```python
from build123d import *

# Parameters (mm, degrees)
SKETCH1_W           = 72
SKETCH1_H           = 42
BOSS_EXTRUDE1_DEPTH = 5
SKETCH2_R           = 1.75
CUT_EXTRUDE1_DEPTH  = 10
D_GAGEMENT_M51_D    = 5.5
SKETCH6_R           = 12.5
CUT_EXTRUDE2_DEPTH  = 42.976183724


with BuildPart() as part:
    # Sketch1 → Boss-Extrude1 (new body)
    with BuildSketch(Plane.XY):
        Rectangle(SKETCH1_W, SKETCH1_H)
    extrude(amount=BOSS_EXTRUDE1_DEPTH)

    # Sketch2 → Cut-Extrude1 (cut)
    with BuildSketch(Plane.XY.offset(5)):
        with Locations((30.475, 15.5)):
            Circle(SKETCH2_R)
        with Locations((30.475, -15.5)):
            Circle(SKETCH2_R)
        with Locations((-0.525, -15.5)):
            Circle(SKETCH2_R)
        with Locations((-0.525, 15.5)):
            Circle(SKETCH2_R)
    extrude(amount=-CUT_EXTRUDE1_DEPTH, mode=Mode.SUBTRACT)

    # Dégagement M51 (through all)
    with Locations(Plane(origin=(0, 0, 0), x_dir=(-1, 0, 0), z_dir=(0, 0, -1))):
        with Locations((21, 11), (21, -11)):
            Hole(D_GAGEMENT_M51_D / 2)

    # Sketch6 → Cut-Extrude2 (cut, through all)
    with BuildSketch(Plane(origin=(0, 0, 0), x_dir=(-1, 0, 0), z_dir=(0, 0, -1))):
        with Locations((-14.975, 0)):
            Circle(SKETCH6_R)
    extrude(amount=-CUT_EXTRUDE2_DEPTH, mode=Mode.SUBTRACT)


solid = part.part
```
Design review of the part built by this model. Coordinates are the model's own, in mm. Coordinates: 2 decimals unless noted, no trailing zeros. Loops run counter-clockwise (first coordinate to the right, second up) from the corner with the lowest first, then second, coordinate; pieces in that order, holes last. Notation, with made-up numbers: M 5.5,-31 L 23.5,-31 A23 ccw 23.5,-23 Z; hole C 36.5,-20.75 d11. An arc over 180 degrees is marked long. One line per question, with ' | ' between items.
(1) We need section A-A (x = -21). Give the boundary of the cut face in (y, z).
Filled in:
outline: M -21,0 L -13.75,0 L -13.75,5 L -21,5 Z; M -8.25,0 L 8.25,0 L 8.25,5 L -8.25,5 Z; M 13.75,0 L 21,0 L 21,5 L 13.75,5 Z
(2) Draft analysis for pull direction X (two halves, no side actions). For faces 1 (the face through (-36, 0, 2)), 2 (the face through (-1, 0, 0)), 3 (the face through (-23.747, -10.879, 2.535)), state which applies: released by +X, released by -X, zero draft, split by the parting line, or undercut.
Filled in:
face 1: released by -X | face 2: zero draft | face 3: undercut
(3) Wall thickness on probe 1 along Y at (x, z) = (-21, 1.7); probe 2 along X at (y, z) = (-16.5, 3.05); probe 3 along X at (y, z) = (-13.5, 1.55): over which ranges is each line inside the solid? List them lowest first.
Filled in:
probe 1: y = -21 to -13.75, -8.25 to 8.25, 13.75 to 21 | probe 2: x = -36 to -1.96, 0.91 to 29.04, 31.91 to 36 | probe 3: x = -36 to -22.15, -19.85 to 36
(4) We need section C-C (z = 1.9). Give the boundary of the cut face in (x, y) (3 decimals), and give its area (3 significant figures).
Filled in:
outline: M -36,-21 L 36,-21 L 36,21 L -36,21 Z; hole C -21,-11 d5.5; hole C -21,11 d5.5; hole C -0.525,-15.5 d3.5; hole C -0.525,15.5 d3.5; hole C 14.975,0 d25; hole C 30.475,-15.5 d3.5; hole C 30.475,15.5 d3.5 | area: 2,450 mm^2
(5) We need section B-B (y = -5.5). Give the boundary of the cut face in (x, z).
Filled in:
outline: M -36,0 L 3.75,0 L 3.75,5 L -36,5 Z; M 26.2,0 L 36,0 L 36,5 L 26.2,5 Z
(6) We need section D-D (y = -11). Give the boundary of the cut face in (x, z).
Filled in:
outline: M -36,0 L -23.75,0 L -23.75,5 L -36,5 Z; M -18.25,0 L 9.04,0 L 9.04,5 L -18.25,5 Z; M 20.91,0 L 36,0 L 36,5 L 20.91,5 Z
(7) For pin 1 Ø5.5 at (x, y) = (-0.525, -15.5) entering from -Z, flat-tipped, find the tip position at first contact; note if it passes through.
Filled in:
pin 1: stops at z = 0
